Build history of the part. All positions in model axes, mm. A direction names the side the tool comes from. Give positions to 0.01 mm unless a question says otherwise; leave off trailing zeros. Loops run counter-clockwise (first coordinate to the right, second up) from the corner with the lowest first, then second, coordinate; pieces in that order, holes last. Notation, with made-up numbers: M 27,68 L 53,68 A21 ccw 53,85 Z; hole C 36.25,56.5 d11. An arc over 180 degrees is marked long. Answer as a JSON object with one key per item and string values. Group by question number.
1. Slice it at A-A (y = 6). List the corners of the cut face in (x, z).
2. Slice it at D-D (x = -6.75). List the corners of the cut face in (y, z), then the cut area to 3 significant figures.
3. Drill centre lines: line 1 along Y through (x, z) = (-0.4, 22.5); line 2 along Z through (x, y) = (-0.7, 6); line 3 along Y through (x, z) = (-3, -2). Where is each one in solid material? Low to high. Write a range as [from, to].
4. Slice it at C-C (z = 6). List the corners of the cut face in (x, y).
5. Slice it at B-B (z = 22.5). List the corners of the cut face in (x, y).
6. Drop flat-ended pins along their axis: pin 1 Ø2 at (y, z) = (6, 22.5) entering from -X; pin 2 Ø6 at (y, z) = (6.5, -15) entering from -X; pin 3 Ø1 at (x, z) = (-8, 4) entering from +Y; pin 4 Ø0.8 at (x, y) = (-5.5, 0.5) entering from -Z. Give the stop position or say it passes through.
7. 3-axis set-ups, long thin cutter, end or side, ignore diameter. For faces 1 (the face through (-5, 1, 10)), 2 (the face through (-5.4, 0.5, -7.5)), 3 (the face through (-2.8, 0.6, 27.5)): which of +Z, -Z, +X, -X, +Y, -Y reach the whole face in a straight line?
Autodesk Inventor part; units mm, degrees
ref_plane "YZ Plane" through (0, 0, 0) normal (1, 0, 0) x (0, 1, 0)
ref_plane "XZ Plane" through (0, 0, 0) normal (0, 1, 0) x (-1, 0, 0)
ref_plane "XY Plane" through (0, 0, 0) normal (0, 0, 1) x (1, 0, 0)
sketch "Náčrt1" plane through (0, 0, 0) normal (0, 0, 1) x (1, 0, 0)
  line L0 (-12, 0) -> (2, 0)
  line L1 (0, 12) -> (0, -2)
  line L2 (0, 0) -> (0, 10)
  line L3 (0, 10) -> (-1, 10)
  line L4 (-1, 10) -> (-1, 1)
  line L5 (-1, 1) -> (-10, 1)
  line L6 (-10, 1) -> (-10, 0)
  line L7 (-10, 0) -> (0, 0)
  dimension "d0" = 10
  dimension "d1" = 1
  dimension "d2" = 9
  dimension "d3" = 9
extrude "Vysunutí1" add sketch "Náčrt1" along normal mid plane 55
sketch "Náčrt2" plane through (-1, 1, 27.5) normal (-1, 0, 0) x (0, 0, 1)
  line L0 (-55, 0) -> (0, 0)
  line L1 (0, 9) -> (0, 0)
  line L2 (-55, 9) -> (0, 9)
  line L3 (-55, 0) -> (-55, 9)
  point P0 (-27.5, -1)
  point P1 (-5, 5)
  dimension "d6" = 5
  dimension "d7" = 5
hole "Díra1" at (-1, 6, 22.5) direction (1, 0, 0) diameter 2.459 end through all
sketch "Náčrt3" plane through (-10, 1, 27.5) normal (0, 1, 0) x (1, 0, 0)
  line L0 (0, 0) -> (0, 55)
  line L1 (9, 0) -> (0, 0)
  line L2 (9, 55) -> (9, 0)
  line L3 (0, 55) -> (9, 55)
  line L4 (0, 55) -> (9, 55)
  line L5 (9, 55) -> (9, 35)
  line L6 (9, 35) -> (0, 35)
  line L7 (0, 35) -> (0, 55)
  point P0 (10, 27.5)
  dimension "d15" = 20
extrude "Vysunutí2" cut sketch "Náčrt3" against normal through all contours L0 L3 L2 L6
properties part number "lift_tab" material "Hliník 6061"
Established:
{
 "1": {"outline": "M -1,-27.5 L 0,-27.5 L 0,21.27 L -1,21.27 Z; M -1,23.73 L 0,23.73 L 0,27.5 L -1,27.5 Z"},
 "2": {"outline": "M 0,-7.5 L 1,-7.5 L 1,27.5 L 0,27.5 Z", "area": "35.0 mm^2"},
 "3": {"line 1": "y = [0, 4.77], [7.23, 10]", "line 2": "z = [-27.5, 21.27], [23.73, 27.5]", "line 3": "y = [0, 1]"},
 "4": {"outline": "M -10,0 L 0,0 L 0,10 L -1,10 L -1,1 L -10,1 Z"},
 "5": {"outline": "M -10,0 L 0,0 L 0,4.77 L -1,4.77 L -1,1 L -10,1 Z; M -1,7.23 L 0,7.23 L 0,10 L -1,10 Z"},
 "6": {"pin 1": "passes through", "pin 2": "stops at x = -1", "pin 3": "stops at y = 1", "pin 4": "stops at z = -7.5"},
 "7": {"face 1": "+Z, -Z, -X, +Y", "face 2": "-Z, -X, +Y, -Y", "face 3": "+Z, +X, -X, +Y, -Y"}
}
